```python
from build123d import *

# Parameters (mm, degrees)
CYLINDER001_R     = 4.5
CYLINDER001_DEPTH = 1
FILLET_R          = 0.9
CYLINDER_R        = 2.95
CYLINDER_DEPTH    = 15


with BuildPart() as fillet_body:
    # Cylinder001 → Cylinder001 (new body)
    with BuildSketch(Plane.XY.offset(14)):
        Circle(CYLINDER001_R)
    extrude(amount=CYLINDER001_DEPTH)

    # Fillet
    fillet_edges = [fillet_body.edges().sort_by_distance(p)[0] for p in [
        (-4.5, 0, 15),
    ]]
    fillet(fillet_edges, radius=FILLET_R)


with BuildPart() as fusion:
    # Cylinder → Cylinder (new body)
    with BuildSketch(Plane.XY):
        Circle(CYLINDER_R)
    extrude(amount=CYLINDER_DEPTH)

    # Fusion: union Fillet body
    add(fillet_body.part)


solid = fusion.part
```
Check sheet for the modelled part. Datum: model origin and axes. Units: mm. A direction names the side the tool comes from. Coordinates: 2 decimals unless noted, no trailing zeros. Loops run counter-clockwise (first coordinate to the right, second up) from the corner with the lowest first, then second, coordinate; pieces in that order, holes last.
1) Sectioned sample at C-C (z = 10.5). Record the boundary of the cut face in (x, y), and give its area (3 significant figures).
2) Sectioned sample at A-A (y = 0). Record the boundary of the cut face in (x, z).
3) Material ranges on probe 1 along Z at (x, y) = (2.25, 2.75); probe 2 along Y at (x, z) = (0, 1.25); probe 3 along X at (y, z) = (-1.5, 1.5), recorded low to high.
4) Gauge pin test, flat end, axial feed: pin 1 (3 mm diameter, centred on x = -1.5, z = 9, fed in from +Y). Record the tip position at first contact, or that the pin passes through.
5) Access from +Z, -Z, +X, -X, +Y, -Y to the whole of each face (thin tool, end or side, straight path). Record for faces 1 (the face through (1, -3, 14)), 2 (the face through (0, 0, 0)).
Check sheet entries:
1. outline: circle Ø5.9 at (0, 0)
1. area: 27.3 mm2
2. outline: (-4.5, 14) - (-2.95, 14) - (-2.95, 0) - (2.95, 0) - (2.95, 14) - (4.5, 14) - (4.5, 14.1) arc R0.9 ccw to (3.6, 15) - (-3.6, 15) arc R0.9 ccw to (-4.5, 14.1) - close
3. probe 1: z = 14 to 15
3. probe 2: y = -2.95 to 2.95
3. probe 3: x = -2.54 to 2.54
4. pin 1: stops at y = 2.95
5. face 1: -Z
5. face 2: -Z, +X, -X, +Y, -Y
